Study the drawing (mm; zero at the part's minimum x, y, z) and answer. Round coordinates to 2 decimals unless told otherwise and drop trailing zeros. Order: outer loops, then holes, each group sorted by start corner. A loop starts at its lowest first (then second) coordinate and runs counter-clockwise, first axis right, second up. Notation, with made-up numbers: (58, -40) - (97, -40) arc R21 cw to (97, -32) - close; hole circle Ø2 at (-26.75, 13). An arc over 180 degrees is marked (long way). Put each result on its own line as item: value. Start each with the question number.
Q1. Section A-A on x = 12.5 is taken. Give the vertices of the cut face in (y, z).
Q2. Section B-B on z = 19 is taken. Give the vertices of the cut face in (x, y).
Q3. Find the intervals of material crossed by line 1 along X through (y, z) = (1.45, 19); line 2 along Z through (x, y) = (12.5, 2); line 3 along Z through (x, y) = (11.5, 1.45), in increasing order. Write a range as from..to.
Q4. This flat-tipped pin is pushed along its axis until it touches: pin 1 Ø1 at (x, z) = (4, 13) entering from -Y. Where does it stop, or does it pass through?
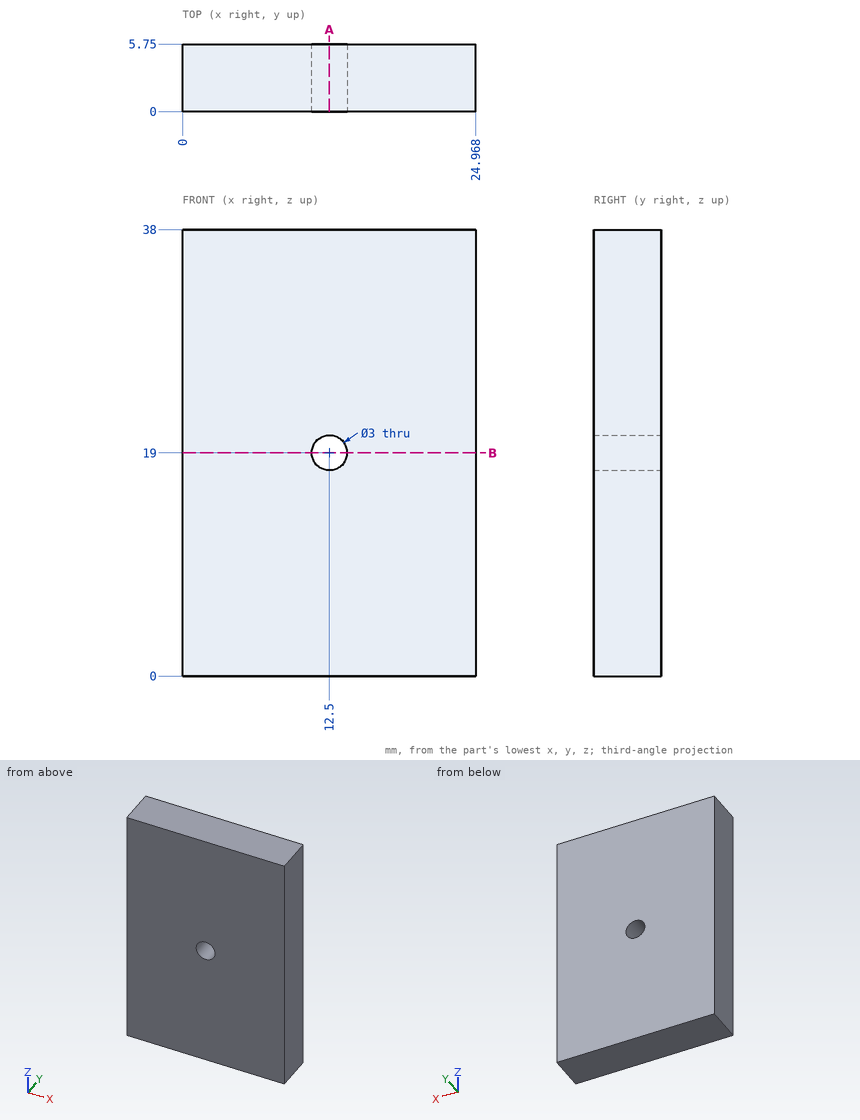
Findings:
1. outline: (0, 0) - (5.75, 0) - (5.75, 17.5) - (0, 17.5) - close; (0, 20.5) - (5.75, 20.5) - (5.75, 38) - (0, 38) - close
2. outline: (0, 0) - (11, 0) - (11, 5.75) - (0, 5.75) - close; (14, 0) - (24.97, 0) - (24.97, 5.75) - (14, 5.75) - close
3. line 1: 0..11, 14..24.97
3. line 2: 0..17.5, 20.5..38
3. line 3: 0..17.88, 20.12..38
4. pin 1: y = 0
